```python
from build123d import *

# Parameters (mm, degrees)
MODEL_R             = 14.351
BOSS_EXTRUDE1_DEPTH = 6.35


with BuildPart() as part:
    # Model → Boss-Extrude1 (new body)
    with BuildSketch(Plane.XY):
        with BuildLine():
            Line((-314.23831963, -55.359484793), (-205.338802982, 104.650248016))
            Line((-205.338802982, 104.650248016), (-11.396613492, 104.650248016))
            Line((-11.396613492, 104.650248016), (-2.138802982, 104.650248016))
            Line((-2.138802982, 104.650248016), (10.561197018, 104.650248016))
            ThreePointArc((10.561197018, 104.650248016), (25.72621731, 99.626267243), (34.892121825, 86.541756641))
            Line((34.892121825, 86.541756641), (46.592108535, 47.500248016))
            ThreePointArc((46.592108535, 47.500248016), (56.051698972, 33.745564192), (71.88314884, 28.450248016))
            Line((71.88314884, 28.450248016), (77.072108535, 28.450248016))
            ThreePointArc((77.072108535, 28.450248016), (95.032620777, 35.889735774), (102.472108535, 53.850248016))
            Line((102.472108535, 53.850248016), (102.472108535, 83.872407327))
            Line((102.472108535, 83.872407327), (102.472108535, 112.853785651))
            ThreePointArc((102.472108535, 112.853785651), (99.24880288, 125.237413065), (90.396972478, 134.478031323))
            Line((90.396972478, 134.478031323), (-199.949582693, 313.389629113))
            ThreePointArc((-199.949582693, 313.389629113), (-219.402189514, 318.224062751), (-236.303247901, 307.447705012))
            Line((-236.303247901, 307.447705012), (-436.377385414, 13.472026599))
            Line((-436.377385414, 13.472026599), (-385.58146606, -51.20282143))
            ThreePointArc((-385.58146606, -51.20282143), (-376.71145599, -58.357541068), (-365.605974805, -60.913979882))
            Line((-365.605974805, -60.913979882), (-324.737451002, -60.913979882))
            ThreePointArc((-324.737451002, -60.913979882), (-318.798508014, -59.439796386), (-314.23831963, -55.359484793))
        make_face()
        with Locations((-323.775189267, -35.513979882)):
            Circle(MODEL_R, mode=Mode.SUBTRACT)
        with Locations((-399.975189267, 2.586020118)):
            Circle(MODEL_R, mode=Mode.SUBTRACT)
        Polygon((77.727371227, 60.200248016), (81.393545437, 53.850248016), (77.727371227, 47.500248016), (70.395022809, 47.500248016), (66.728848599, 53.850248016), (70.395022809, 60.200248016), align=None, mode=Mode.SUBTRACT)
        with Locations((-190.707148919, 138.516914683)):
            Circle(MODEL_R, mode=Mode.SUBTRACT)
        with Locations((-208.832932893, 283.437784316)):
            Circle(MODEL_R, mode=Mode.SUBTRACT)
    extrude(amount=BOSS_EXTRUDE1_DEPTH)


solid = part.part
```
Part model, mm, in its own coordinate system. A direction names the side the tool comes from. Round coordinates to 2 decimals unless told otherwise and drop trailing zeros. Write each loop counter-clockwise with the first axis right and the second up, starting at its lowest first coordinate (ties: lowest second). Pieces come first, ordered by that corner, then holes.
Item 1: Drop flat-ended pins along their axis: pin 1 Ø3 at (x, z) = (-95, 4.5) entering from -Y; pin 2 Ø2 at (y, z) = (150.5, 5) entering from -X; pin 3 Ø1.9 at (x, z) = (75.5, 2.5) entering from +Y. Give the stop position or say it passes through.
Results:
pin 1: stops at y = 104.65
pin 2: stops at x = -343.8
pin 3: stops at y = 144.24
Item 2: Two-plate mould, pull along Y, no slides. Class faces 3 (the flat face through (-171, 131, 0)), 4 (the cylindrical face through (-210.701, 297.667, 3.131)), 5 (the cylindrical face through (-219.12, 318.27, 3.13)): +Y half, -Y half, draft (parallel to the pull), parting line (faces both ways), or undercut.
Results:
face 3: draft
face 4: undercut
face 5: +Y half
Item 3: Cut at B-B, the plane y = 250. Give the cut face in (x, z).
Results:
outline: (-275.4, 0) - (-97.08, 0) - (-97.08, 6.35) - (-275.4, 6.35) - close
Item 4: Which spindle directions (+Z, -Z, +X, -X, +Y, -Y) get a long thin tool onto all of the face, cutting with end or side? Do faces 1 (the flat face through (-260.55, 23.53, 3.13)), 2 (the flat face through (-52.74, 222.68, 3.13)). Say none if no direction does.
Results:
face 1: +Z, -Z, -Y
face 2: +Z, -Z, +X, +Y
Item 5: Probe L1, parallel to X at y = -40, z = 4.5; L2, parallel to X at y = 149, z = 3.25; L3, parallel to Y at x = -344.5, z = 4.25. List the from-to ranges inside material, lowest first.
Results:
L1: x = -394.38 to -337.41, -310.14 to -303.78
L2: x = -344.14 to -200.51, -180.91 to 66.83
L3: y = -60.91 to 148.47
Item 6: Cut at A-A, the plane z = 2.75. Give the cut face in (x, y).
Results:
outline: (-436.38, 13.47) - (-385.58, -51.2) arc R25.4 ccw to (-365.61, -60.91) - (-324.74, -60.91) arc R12.7 ccw to (-314.24, -55.36) - (-205.34, 104.65) - (10.56, 104.65) arc R25.4 cw to (34.89, 86.54) - (46.59, 47.5) arc R26.31 ccw to (71.88, 28.45) - (77.07, 28.45) arc R25.4 ccw to (102.47, 53.85) - (102.47, 112.85) arc R25.4 ccw to (90.4, 134.48) - (-199.95, 313.39) arc R25.4 ccw to (-236.3, 307.45) - close; hole circle Ø28.7 at (-399.98, 2.59); hole circle Ø28.7 at (-323.78, -35.51); hole circle Ø28.7 at (-208.83, 283.44); hole circle Ø28.7 at (-190.71, 138.52); hole (66.73, 53.85) - (70.4, 47.5) - (77.73, 47.5) - (81.39, 53.85) - (77.73, 60.2) - (70.4, 60.2) - close
Item 7: Cut at C-C, the plane x = -103. Give the cut face in (y, z).
Results:
outline: (104.65, 0) - (253.65, 0) - (253.65, 6.35) - (104.65, 6.35) - close
